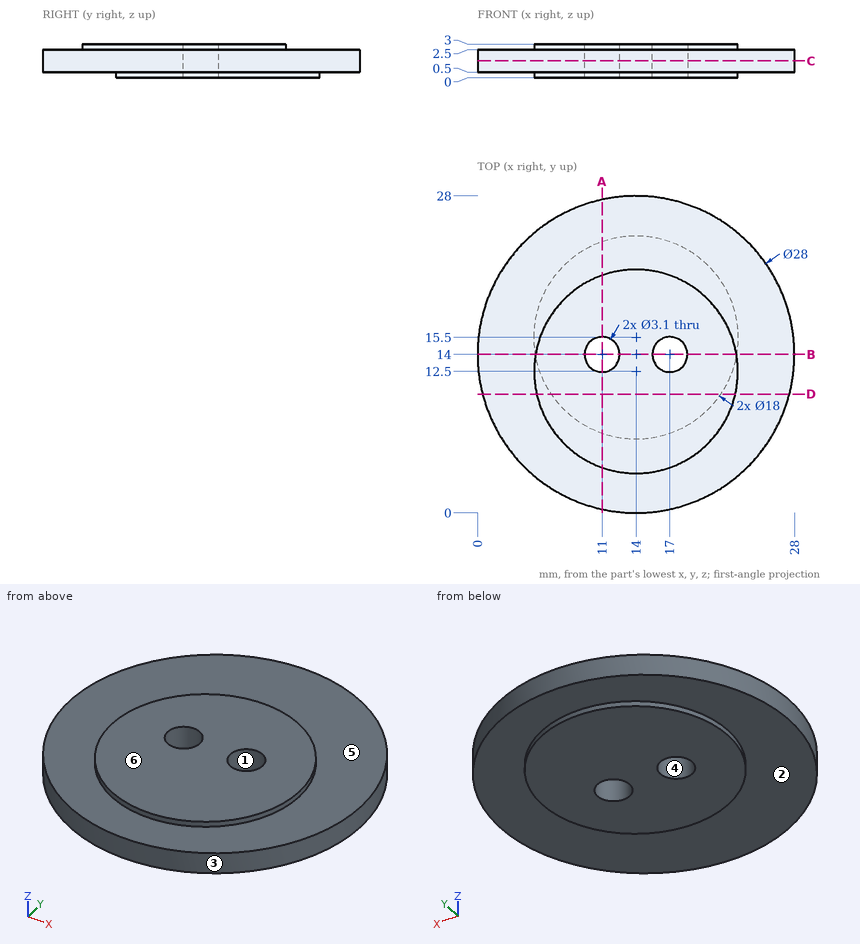
Job drawing, mm, ordinate dimensions from the low corner. One solid piece. A direction names the side the tool comes from. Coordinates: 2 decimals unless noted, no trailing zeros. Order: outer loops, then holes, each group sorted by start corner. A loop starts at its lowest first (then second) coordinate and runs counter-clockwise, first axis right, second up. Notation, with made-up numbers: (7, 13) - (40, 13) arc R22 ccw to (40, 25) - close; hole circle Ø11 at (20, 35). An arc over 180 degrees is marked (long way). Use CSV: the item, a comma, the result in double quotes.
Item 1: Saw through at D-D on y = 10.5. Give the cut face in (x, z).
Solved:
outline,"(0.44, 0.5) - (6.52, 0.5) - (6.52, 0) - (21.48, 0) - (21.48, 0.5) - (27.56, 0.5) - (27.56, 2.5) - (22.77, 2.5) - (22.77, 3) - (5.23, 3) - (5.23, 2.5) - (0.44, 2.5) - close"
Item 2: 3-axis set-ups, long thin cutter, end or side, ignore diameter. For the marked faces 5 and 6: which of +Z, -Z, +X, -X, +Y, -Y reach the whole face in a straight line?
Solved:
face 5,"+Z"
face 6,"+Z, +X, -X, +Y, -Y"
Item 3: Saw through at C-C on z = 1.5. Give the cut face in (x, y), and give its area (3 significant figures).
Solved:
outline,"circle Ø28 at (14, 14); hole circle Ø3.1 at (11, 14); hole circle Ø3.1 at (17, 14)"
area,"601 mm²"
Item 4: Drop flat-ended pins along their axis: P1, Ø1, axis at x = 23.5, y = 6.5, coming from the -Z side; P2, Ø1.5, axis at x = 9.5, z = 2.5, coming from the +Y side; P3, Ø1, axis at x = 9, z = 2.5, coming from the -Y side. Give the stop position or say it passes through.
Solved:
P1,"stops at z = 0.5"
P2,"stops at y = 27.49"
P3,"stops at y = 0.74"
Item 5: Saw through at A-A on x = 11. Give the cut face in (y, z), and give its area (3 significant figures).
Solved:
outline,"(0.33, 0.5) - (7.01, 0.5) - (7.01, 0) - (12.45, 0) - (12.45, 3) - (4.01, 3) - (4.01, 2.5) - (0.33, 2.5) - close; (15.55, 0) - (23.99, 0) - (23.99, 0.5) - (27.67, 0.5) - (27.67, 2.5) - (20.99, 2.5) - (20.99, 3) - (15.55, 3) - close"
area,"62.4 mm²"
Item 6: Saw through at B-B on y = 14. Give the cut face in (x, z).
Solved:
outline,"(0, 0.5) - (5.13, 0.5) - (5.13, 0) - (9.45, 0) - (9.45, 3) - (5.13, 3) - (5.13, 2.5) - (0, 2.5) - close; (12.55, 0) - (15.45, 0) - (15.45, 3) - (12.55, 3) - close; (18.55, 0) - (22.87, 0) - (22.87, 0.5) - (28, 0.5) - (28, 2.5) - (22.87, 2.5) - (22.87, 3) - (18.55, 3) - close"
Item 7: Probe probe 1 along X at (y, z) = (14.75, 2); probe 2 along Y at (x, z) = (17, 1.7); probe 3 along Z at (x, y) = (8.5, 24.5). List the from-to ranges inside material, lowest first.
Solved:
probe 1,"x = 0.02 to 9.64, 12.36 to 15.64, 18.36 to 27.98"
probe 2,"y = 0.33 to 12.45, 15.55 to 27.67"
probe 3,"z = 0.5 to 2.5"
Item 8: Mould opens along Y. For the marked faces 1, 2, 3 and 4 say: +Y half, -Y half, draft (parallel to the pull), parting line (faces both ways), or undercut.
Solved:
face 1,"undercut"
face 2,"draft"
face 3,"parting line"
face 4,"undercut"
